The listing builds one solid part. Answer for the finished solid, in the listing's coordinates (mm). A direction names the side the tool comes from. Give positions to 0.01 mm unless a question says otherwise; leave off trailing zeros. Write each loop counter-clockwise with the first axis right and the second up, starting at its lowest first coordinate (ties: lowest second). Pieces come first, ordered by that corner, then holes. Notation, with made-up numbers: M -28,31.5 L -15,31.5 A16 ccw -15,39.5 Z; hole C 46,59.5 d10. An arc over 180 degrees is marked long. Return JSON: item names as keys, results as strings.
from build123d import *

# Parameters (mm, degrees)
PAD_DEPTH    = 60
POCKET_DEPTH = 21.9353755374


with BuildPart() as part:
    # Sketch → Pad (new body)
    with BuildSketch(Plane.XY):
        with BuildLine():
            Line((-4.0957602214, -5.8493517964), (-34.4145861811, -49.1491226573))
            Line((-34.4145861811, -49.1491226573), (-45.473138779, -41.4058407666))
            Line((-45.473138779, -41.4058407666), (-42.6052565972, -37.3100805452))
            Line((-42.6052565972, -37.3100805452), (-44.2435606858, -36.1629276725))
            ThreePointArc((-44.2435606858, -36.1629276725), (-44.9907852998, -35.9972719637), (-45.6362891664, -36.4085032804))
            Line((-45.6362891664, -36.4085032804), (-49.0777477845, -41.3234155461))
            ThreePointArc((-49.0777477845, -41.3234155461), (-49.2434034933, -42.0706401601), (-48.8321721766, -42.7161440268))
            Line((-48.8321721766, -42.7161440268), (-34.4970114015, -52.7537316629))
            ThreePointArc((-34.4970114015, -52.7537316629), (-33.7497867875, -52.9193873716), (-33.1042829209, -52.508156055))
            Line((-33.1042829209, -52.508156055), (-8.1915204429, -16.9290439796))
            ThreePointArc((8.1915204429, -16.9290439796), (0, -12.6648083431), (-8.1915204429, -16.9290439796))
            Line((8.1915204429, -16.9290439796), (29.1048677003, -46.7963991796))
            ThreePointArc((20.9133472575, -62.5321635431), (29.7834555892, -57.1496496755), (29.1048677003, -46.7963991796))
            Line((20.9133472575, -62.5321635431), (-42.1138850919, -62.5321635431))
            ThreePointArc((-42.1138850919, -62.5321635431), (-43.5280986543, -63.1179499807), (-44.1138850919, -64.5321635431))
            Line((-44.1138850919, -64.5321635431), (-44.1138850919, -65.5321635431))
            Line((-44.1138850919, -65.5321635431), (36.2812042732, -65.5321635431))
            ThreePointArc((36.2812042732, -65.5321635431), (40.7162584391, -62.8409066093), (40.3769644947, -57.6642813614))
            Line((40.3769644947, -57.6642813614), (4.0957602214, -5.8493517964))
            ThreePointArc((4.0957602214, -5.8493517964), (0, -3.7172339781), (-4.0957602214, -5.8493517964))
        make_face()
    extrude(amount=PAD_DEPTH)

    # Sketch001 (on Face9 of Pad) → Pocket (cut, through all)
    with BuildSketch(Plane(origin=(-34.4145861811, -49.1491226573, 0), x_dir=(-0.8191520443, 0.5735764364, 0), z_dir=(0.5735764364, 0.8191520443, 0))):
        with BuildLine():
            Line((1.75, 24.5), (1.75, 35.5))
            ThreePointArc((3.25, 37), (2.1893398282, 36.5606601718), (1.75, 35.5))
            Line((3.25, 37), (10.25, 37))
            ThreePointArc((11.75, 35.5), (11.3106601718, 36.5606601718), (10.25, 37))
            Line((11.75, 35.5), (11.75, 24.5))
            ThreePointArc((10.25, 23), (11.3106601718, 23.4393398282), (11.75, 24.5))
            Line((10.25, 23), (3.25, 23))
            ThreePointArc((1.75, 24.5), (2.1893398282, 23.4393398282), (3.25, 23))
        make_face()
    extrude(amount=-POCKET_DEPTH, mode=Mode.SUBTRACT)


solid = part.part
Item 1: Determine the mould class of faces 6 (the flat face through (-4, -65.532, 30)), 7 (the flat face through (-37, -51, 30)), 8 (the flat face through (22.49, -32.12, 29.58)), 9 (the cylindrical face through (0.134, -12.666, 29.58)) for opening direction Y: +Y half, -Y half, draft (parallel to the pull), parting line (faces both ways), or undercut.
Geometry results:
{"face 6": "-Y half", "face 7": "undercut", "face 8": "+Y half", "face 9": "undercut"}
Item 2: Which of the six approach directions +Z, -Z, +X, -X, +Y, -Y give full straight-line access (tool end or side, diameter ignored) to faces 1 (the cylindrical face through (29.712, -57.285, 29.58)), 2 (the cylindrical face through (-37.05, -49.11, 23.45)), 3 (the flat face through (-10, -62.532, 30)), 4 (the flat face through (-19.043, -27.196, 29.58)), 5 (the cylindrical face through (-44.54, -43.87, 36.55))?
Geometry results:
{"face 1": "+Z, -Z", "face 2": "-X, +Y", "face 3": "+Z, -Z, -X", "face 4": "+Z, -Z, +Y", "face 5": "none"}
Item 3: Given pin 1 Ø8 at (x, z) = (-7.5, 33) entering from +Y; pin 2 Ø10 at (x, y) = (-3, -57.5) entering from +Z; pin 3 Ø6 at (y, z) = (-46, 19) entering from +X; pin 4 Ø2 at (y, z) = (-51.5, 33) entering from +X, each flat-ended and moving along its own axis, determine where each tip first touches the part or whether it passes through.
Geometry results:
{"pin 1": "stops at y = -5.15", "pin 2": "passes through", "pin 3": "stops at x = 34.31", "pin 4": "stops at x = 36.76"}
Item 4: A cutting plane is placed at B-B, the plane z = 16.5. Write down the section's boundary in (x, y), plus the area to 3 significant figures.
Geometry results:
{"outline": "M -49.08,-41.32 A1 ccw -48.83,-42.72 L -34.5,-52.75 A1 ccw -33.1,-52.51 L -8.19,-16.93 A10 cw 8.19,-16.93 L 29.1,-46.8 A10 cw 20.91,-62.53 L -42.11,-62.53 A2 ccw -44.11,-64.53 L -44.11,-65.53 L 36.28,-65.53 A5 ccw 40.38,-57.66 L 4.1,-5.85 A5 ccw -4.1,-5.85 L -34.41,-49.15 L -45.47,-41.41 L -42.61,-37.31 L -44.24,-36.16 A1 ccw -45.64,-36.41 Z", "area": "829 mm2"}
Item 5: A cutting plane is placed at C-C, the plane x = 16. Write down the section's boundary in (y, z), plus the area to 3 significant figures.
Geometry results:
{"outline": "M -65.53,0 L -62.53,0 L -62.53,60 L -65.53,60 Z; M -28.08,0 L -22.85,0 L -22.85,60 L -28.08,60 Z", "area": "494 mm2"}
Item 6: Find the intervals of material crossed by line 1 (X direction, y = -44, z = 6.5); line 2 (X direction, y = -40.5, z = 9); line 3 (Y direction, x = 9.5, z = 38.5), in increasing order.
Geometry results:
{"line 1": "x = -47 to -41.77, -30.81 to -27.15, 27.15 to 30.81", "line 2": "x = -48.5 to -44.84, -28.36 to -24.7, 24.7 to 28.36", "line 3": "y = -65.53 to -62.53, -18.8 to -13.57"}
Item 7: A cutting plane is placed at D-D, the plane x = 35. Write down the section's boundary in (y, z), plus the area to 3 significant figures.
Geometry results:
{"outline": "M -65.53,0 L -49.99,0 L -49.99,60 L -65.53,60 Z", "area": "933 mm2"}
Item 8: A cutting plane is placed at A-A, the plane y = -25. Write down the section's boundary in (x, z).
Geometry results:
{"outline": "M -17.51,0 L -13.84,0 L -13.84,60 L -17.51,60 Z; M 13.84,0 L 17.51,0 L 17.51,60 L 13.84,60 Z"}
